Design review of the part built by this model. Coordinates are the model's own, in mm. A direction names the side the tool comes from. Give positions to 0.01 mm unless a question says otherwise; leave off trailing zeros. Write each loop counter-clockwise with the first axis right and the second up, starting at its lowest first coordinate (ties: lowest second). Pieces come first, ordered by that corner, then holes. Notation, with made-up numbers: (21.5, 49.25) - (68.5, 49.25) arc R30 cw to (68.5, 81.25) - close; hole circle Ø5 at (-32.75, 78.5). An arc over 180 degrees is marked (long way). Use a Markdown table: item, result. Add a question column.
```python
from build123d import *

# Parameters (mm, degrees)
F0_W          = 5.08
F0_H          = 9.99998
F1_DEPTH      = 12.5
F2_W          = 9.99998
F2_H          = 7.42
F3_DEPTH      = 2.54
F4_W          = 9.99998
F4_H          = 7.42
F5_DEPTH      = 2.54
F6_W          = 2.54
F6_H          = 9.99998
F7_DEPTH      = 5.08
F8_W          = 10.16
F8_H          = 2.032
F9_DEPTH      = 5.08
F9_DEPTH_BACK = 7.62
F10_T1_DEPTH  = 30.48
F11_R         = 1.27
F12_T1_DEPTH  = 22.6034078934


# Not quite as in the source:
# - a fillet or chamfer that OpenCascade refuses, or shapes differently, is made with other operations: its cross-section is extruded or revolved along the edge and cut away or added


with BuildPart() as f1:
    # F0 (on Top) → F1 (new body)
    with BuildSketch(Plane.XY):
        with Locations((2.54, 4.99999)):
            Rectangle(F0_W, F0_H)
    extrude(amount=F1_DEPTH)

    # F2 (on face) → F3 (join)
    with BuildSketch(Plane(origin=(0, 0, 0), x_dir=(0, -1, 0), z_dir=(-1, 0, 0))):
        with Locations((-4.99999, 8.79)):
            Rectangle(F2_W, F2_H)
    extrude(amount=F3_DEPTH)

    # F4 (on face) → F5 (join)
    with BuildSketch(Plane.YZ.offset(5.08)):
        with Locations((4.99999, 8.79)):
            Rectangle(F4_W, F4_H)
    extrude(amount=F5_DEPTH)

    # F6 (on face) → F7 (join)
    with BuildSketch(Plane.XY.offset(12.5)):
        with Locations((-1.27, 4.99999)):
            Rectangle(F6_W, F6_H)
        with Locations((6.35, 4.99999)):
            Rectangle(F6_W, F6_H)
    extrude(amount=F7_DEPTH)

    # F8 (on face) → F9 (join, two sides)
    with BuildSketch(Plane(origin=(0, 0, 0), x_dir=(1, 0, 0), z_dir=(0, 0, -1))) as f9_sk:
        with Locations((2.54, 1.016)):
            Rectangle(F8_W, F8_H)
        with Locations((2.54, -11.01598)):
            Rectangle(F8_W, F8_H)
    extrude(amount=F9_DEPTH)
    extrude(f9_sk.sketch, amount=-F9_DEPTH_BACK)

    # F10: fillet of radius 5.08 on 2 edges, made by hand

    # F10_s2 → F10_t1 (cut)
    with BuildSketch(Plane.YZ.offset(-12.7)):
        with BuildLine():
            ThreePointArc((0, 7.62), (-1.4956901303, 5.8278450651), (-2.032, 3.556))
            Line((-2.032, 3.556), (-2.032, 7.62))
            Line((-2.032, 7.62), (0, 7.62))
        make_face()
        with BuildLine():
            ThreePointArc((12.03198, 3.556), (11.4956701303, 5.8278450651), (9.99998, 7.62))
            Line((9.99998, 7.62), (12.03198, 7.62))
            Line((12.03198, 7.62), (12.03198, 3.556))
        make_face()
    extrude(amount=F10_T1_DEPTH, mode=Mode.SUBTRACT)

    # F11
    f11_edges = [f1.edges().sort_by_distance(p)[0] for p in [
        (-1.27, 0, 17.58),
        (6.35, 0, 17.58),
        (6.35, 9.99998, 17.58),
        (-1.27, 9.99998, 17.58),
    ]]
    fillet(f11_edges, radius=F11_R)

    # F12: fillet of radius 2.54 on 2 edges, made by hand

    # F12_s2 → F12_t1 (cut)
    with BuildSketch(Plane.YZ.offset(-8.7617039467)):
        with BuildLine():
            ThreePointArc((-2.032, -2.5913184213), (-1.4594755399, -4.1977554727), (0, -5.08))
            Line((0, -5.08), (-2.032, -5.08))
            Line((-2.032, -5.08), (-2.032, -2.5913184213))
        make_face()
        with BuildLine():
            ThreePointArc((12.03198, -2.5913184213), (11.4594555399, -4.1977554727), (9.99998, -5.08))
            Line((9.99998, -5.08), (12.03198, -5.08))
            Line((12.03198, -5.08), (12.03198, -2.5913184213))
        make_face()
    extrude(amount=F12_T1_DEPTH, mode=Mode.SUBTRACT)


solid = f1.part
```
(1) Add section C-C (x = 7). State the section outline as (y, z) points.
(2) Add section D-D (y = 7.25). State the section outline as (x, z) points.
(3) Insertion check: pin 1 (3 mm diameter, centred on y = 2, z = 0, fed in from +X); pin 2 (6 mm diameter, centred on x = -0.5, z = 12, fed in from +Y); pin 3 (2.5 mm diameter, centred on x = 1, z = 10.5, fed in from -Y). Each pin has a flat end and moves straight along its axis. Give the tip position at first contact, or say it passes through.
(4) For line 1 along X through (y, z) = (4, 15.75); line 2 along Y through (x, z) = (6.5, 12); line 3 along X through (y, z) = (2.5, 3.5), list the stretches that pass through material, from the lowest coordinate up.
(5) Mouldability with a two-part tool opening along Y and no side actions: class faces 1 (the face through (5.08, 5, 3)), 2 (the face through (2, -2.032, 0)), 3 (the face through (5.08, 5, 15)) as +Y half, -Y half, draft (parallel to the pull), parting line (faces both ways), or undercut.
(6) Tool access review of faces 4 (the face through (6, 5, 5.08)), 5 (the face through (2, 10, -1)), 6 (the face through (3, 5, 0)): name each direction out of +Z, -Z, +X, -X, +Y, -Y from which nothing blocks a thin tool from reaching the whole face with its end or side.
(7) Add section A-A (z = 15.5). State the section outline as (x, y) points, and give its area (3 significant figures).
(8) Add section B-B (z = -1.5). State the section outline as (x, y) points, and give its area (3 significant figures).
Answers follow:
| question | item | result |
|---|---|---|
| 1 | outline | (-2.03, -2.59) arc R2.54 ccw to (0, -5.08) - (0, 5.08) - (10, 5.08) - (10, -5.08) arc R2.54 ccw to (12.03, -2.59) - (12.03, 3.56) arc R5.08 ccw to (10, 7.62) - (10, 16.31) arc R1.27 ccw to (8.73, 17.58) - (1.27, 17.58) arc R1.27 ccw to (0, 16.31) - (0, 7.62) arc R5.08 ccw to (-2.03, 3.56) - close |
| 2 | outline | (-2.54, 5.08) - (0, 5.08) - (0, 0) - (5.08, 0) - (5.08, 5.08) - (7.62, 5.08) - (7.62, 17.58) - (5.08, 17.58) - (5.08, 12.5) - (0, 12.5) - (0, 17.58) - (-2.54, 17.58) - close |
| 3 | pin 1 | x = 5.08 |
| 3 | pin 2 | y = 10 |
| 3 | pin 3 | y = 0 |
| 4 | line 1 | -2.54 to 0, 5.08 to 7.62 |
| 4 | line 2 | 0 to 10 |
| 4 | line 3 | 0 to 5.08 |
| 5 | face 1 | undercut |
| 5 | face 2 | -Y half |
| 5 | face 3 | draft |
| 6 | face 4 | -Z, +X |
| 6 | face 5 | -Z |
| 6 | face 6 | -Z, +X, -X |
| 7 | outline | (-2.54, 0) - (0, 0) - (0, 10) - (-2.54, 10) - close; (5.08, 0) - (7.62, 0) - (7.62, 10) - (5.08, 10) - close |
| 7 | area | 50.8 mm^2 |
| 8 | outline | (-2.54, -2.03) - (7.62, -2.03) - (7.62, 0) - (-2.54, 0) - close; (-2.54, 10) - (7.62, 10) - (7.62, 12.03) - (-2.54, 12.03) - close |
| 8 | area | 41.3 mm^2 |
